Geometry check sheet. Reference: the model listing, model coordinates, mm. A direction names the side the tool comes from. Round coordinates to 2 decimals unless told otherwise and drop trailing zeros. Order: outer loops, then holes, each group sorted by start corner. A loop starts at its lowest first (then second) coordinate and runs counter-clockwise, first axis right, second up.
(1) Set-up check for faces 1 (the face through (699.988, 66.401, 35.444)), 2 (the face through (893, 67, 23.5)), 3 (the face through (1800, 68, -28)): record each of +Z, -Z, +X, -X, +Y, -Y from which the full face is reachable in a straight line by a thin tool's end or side.
(2) Sectioned sample at A-A (x = 559.5). Record the boundary of the cut face in (y, z).
(3) Material ranges on line 1 along Z through (x, y) = (1232, 63); line 2 along Y through (x, z) = (1098, -3); line 3 along Z through (x, y) = (113, -15), recorded low to high.
(4) Go/stop test with flat-tipped pins: pin 1 (2 mm diameter, centred on x = 719.5, y = 91, fed in from +Z); pin 2 (1.5 mm diameter, centred on x = 929.5, z = 2.5, fed in from -Y); pin 3 (10 mm diameter, centred on x = 1400, z = 27, fed in from +Y). Record where each tip stops, or that it passes through.
(5) Release check for a two-part mould opening along X. For faces 4 (the face through (1731, 42, 39.5)), 5 (the face through (135.015, -19.34, -35.444)), 6 (the face through (14.121, 68.485, -35.444)) record: +X half, -X half, draft (parallel to the pull), parting line (faces both ways), or undercut.
(6) Sectioned sample at C-C (x = 1185.5). Record the boundary of the cut face in (y, z).
from build123d import *

# Parameters (mm, degrees)
SKETCH3_W           = 63
SKETCH3_H           = 100
SKETCH3_W_2         = 47
SKETCH3_H_2         = 84
BOSS_EXTRUDE1_DEPTH = 1800
FILLET1_R           = 15
SKETCH4_R           = 15
BOSS_EXTRUDE2_DEPTH = 8
CUT_EXTRUDE3_DEPTH  = 80
CUT_EXTRUDE5_DEPTH  = 63
SKETCH8_R           = 15
BOSS_EXTRUDE3_DEPTH = 8
CUT_EXTRUDE6_DEPTH  = 80.0000001


with BuildPart() as part:
    # Sketch3 → Boss-Extrude1 (new body)
    with BuildSketch(Plane(origin=(0, 0, 0), x_dir=(0, 0, -1), z_dir=(1, 0, 0))):
        with Locations((0, 67.5)):
            Rectangle(SKETCH3_W, SKETCH3_H)
        with Locations((0, 67.5)):
            Rectangle(SKETCH3_W_2, SKETCH3_H_2, mode=Mode.SUBTRACT)
    extrude(amount=BOSS_EXTRUDE1_DEPTH)

    # Fillet1
    fillet1_edges = [part.edges().sort_by_distance(p)[0] for p in [
        (900, 109.5, 23.5),
        (900, 25.5, 23.5),
        (900, 25.5, -23.5),
        (900, 109.5, -23.5),
        (900, 17.5, -31.5),
        (900, 17.5, 31.5),
        (900, 117.5, 31.5),
        (900, 117.5, -31.5),
    ]]
    fillet(fillet1_edges, radius=FILLET1_R)

    # Sketch4 → Boss-Extrude2 (add)
    with BuildSketch(Plane.XY.offset(31.5)):
        with BuildLine():
            Line((51.132453633, 117.5), (-23.941241068, 18.07807999))
            ThreePointArc((-23.941241068, 18.07807999), (-27.681309785, -11.564821166), (-3.964911603, -29.73683702))
            Line((-3.964911603, -29.73683702), (146.035088397, -49.73683702))
            ThreePointArc((146.035088397, -49.73683702), (152.009214612, -49.932641992), (157.903578304, -48.940170179))
            Line((157.903578304, -48.940170179), (375.312967218, 10.434467861))
            ThreePointArc((375.312967218, 10.434467861), (401.42242053, 15.725747031), (428.003489242, 17.5))
            Line((428.003489242, 17.5), (650, 17.5))
            ThreePointArc((650, 17.5), (700, 67.5), (650, 117.5))
            Line((650, 117.5), (51.132453633, 117.5))
        make_face()
        Circle(SKETCH4_R, mode=Mode.SUBTRACT)
        with Locations((150, -20)):
            Circle(SKETCH4_R, mode=Mode.SUBTRACT)
    boss_extrude2 = extrude(amount=BOSS_EXTRUDE2_DEPTH)

    # Mirror2: Boss-Extrude2 across plane
    add(boss_extrude2.mirror(Plane.XY))

    # Sketch5 → Cut-Extrude3 (cut, through all)
    with BuildSketch(Plane.XY.offset(39.5)):
        with BuildLine():
            Line((290.508026136, 96.142023945), (345.508026136, 96.142023945))
            ThreePointArc((345.508026136, 96.142023945), (365.508026136, 76.142023945), (345.508026136, 56.142023945))
            Line((345.508026136, 56.142023945), (290.508026136, 56.142023945))
            ThreePointArc((290.508026136, 56.142023945), (270.508026136, 76.142023945), (290.508026136, 96.142023945))
        make_face()
    extrude(amount=-CUT_EXTRUDE3_DEPTH, mode=Mode.SUBTRACT)

    # Sketch7 → Cut-Extrude5 (cut)
    with BuildSketch(Plane.XY.offset(31.5)):
        Polygon((0, 17.5), (51.132453633, 117.5), (-2.794234501, 117.5), (-2.794234501, 17.5), align=None)
    extrude(amount=-CUT_EXTRUDE5_DEPTH, mode=Mode.SUBTRACT)

    # Sketch8 → Boss-Extrude3 (add)
    with BuildSketch(Plane.XY.offset(31.5)):
        with BuildLine():
            Line((1573.208774734, 17.5), (1714.67806612, 17.5))
            ThreePointArc((1714.67806612, 17.5), (1798.428366058, -3.186841446), (1862.91487867, -60.489091313))
            ThreePointArc((1862.91487867, -60.489091313), (1918.389175604, -76.071136101), (1943.712509929, -24.312789154))
            ThreePointArc((1943.712509929, -24.312789154), (1877.887370152, 77.812206283), (1763.051214044, 117.5))
            Line((1763.051214044, 117.5), (1573.208774734, 117.5))
            ThreePointArc((1573.208774734, 117.5), (1523.208774734, 67.5), (1573.208774734, 17.5))
        make_face()
        with Locations((1900, -35)):
            Circle(SKETCH8_R, mode=Mode.SUBTRACT)
    boss_extrude3 = extrude(amount=BOSS_EXTRUDE3_DEPTH)

    # Mirror8: Boss-Extrude3 across plane
    add(boss_extrude3.mirror(Plane.XY))

    # Sketch9 → Cut-Extrude6 (cut, through all)
    with BuildSketch(Plane.XY.offset(39.5)):
        with BuildLine():
            Line((1668.198215583, 87.5), (1733.198215583, 87.5))
            ThreePointArc((1733.198215583, 87.5), (1753.198215583, 67.5), (1733.198215583, 47.5))
            Line((1733.198215583, 47.5), (1668.198215583, 47.5))
            ThreePointArc((1668.198215583, 47.5), (1648.198215583, 67.5), (1668.198215583, 87.5))
        make_face()
    extrude(amount=-CUT_EXTRUDE6_DEPTH, mode=Mode.SUBTRACT)


solid = part.part
Answer below:
1. face 1: +Z
1. face 2: +X, -X
1. face 3: +X, +Y, -Y
2. outline: (17.5, -39.5) - (117.5, -39.5) - (117.5, -31.5) - (102.5, -31.5) arc R15 ccw to (117.5, -16.5) - (117.5, 16.5) arc R15 ccw to (102.5, 31.5) - (117.5, 31.5) - (117.5, 39.5) - (17.5, 39.5) - (17.5, 31.5) - (32.5, 31.5) arc R15 ccw to (17.5, 16.5) - (17.5, -16.5) arc R15 ccw to (32.5, -31.5) - (17.5, -31.5) - close; hole (25.5, -8.5) arc R15 ccw to (40.5, -23.5) - (94.5, -23.5) arc R15 ccw to (109.5, -8.5) - (109.5, 8.5) arc R15 ccw to (94.5, 23.5) - (40.5, 23.5) arc R15 ccw to (25.5, 8.5) - close
3. line 1: z = -31.5 to -23.5, 23.5 to 31.5
3. line 2: y = 17.5 to 25.5, 109.5 to 117.5
3. line 3: z = -39.5 to -31.5, 31.5 to 39.5
4. pin 1: stops at z = 31.5
4. pin 2: stops at y = 17.5
4. pin 3: stops at y = 116.46
5. face 4: draft
5. face 5: undercut
5. face 6: -X half
6. outline: (17.5, -16.5) arc R15 ccw to (32.5, -31.5) - (102.5, -31.5) arc R15 ccw to (117.5, -16.5) - (117.5, 16.5) arc R15 ccw to (102.5, 31.5) - (32.5, 31.5) arc R15 ccw to (17.5, 16.5) - close; hole (25.5, -8.5) arc R15 ccw to (40.5, -23.5) - (94.5, -23.5) arc R15 ccw to (109.5, -8.5) - (109.5, 8.5) arc R15 ccw to (94.5, 23.5) - (40.5, 23.5) arc R15 ccw to (25.5, 8.5) - close
